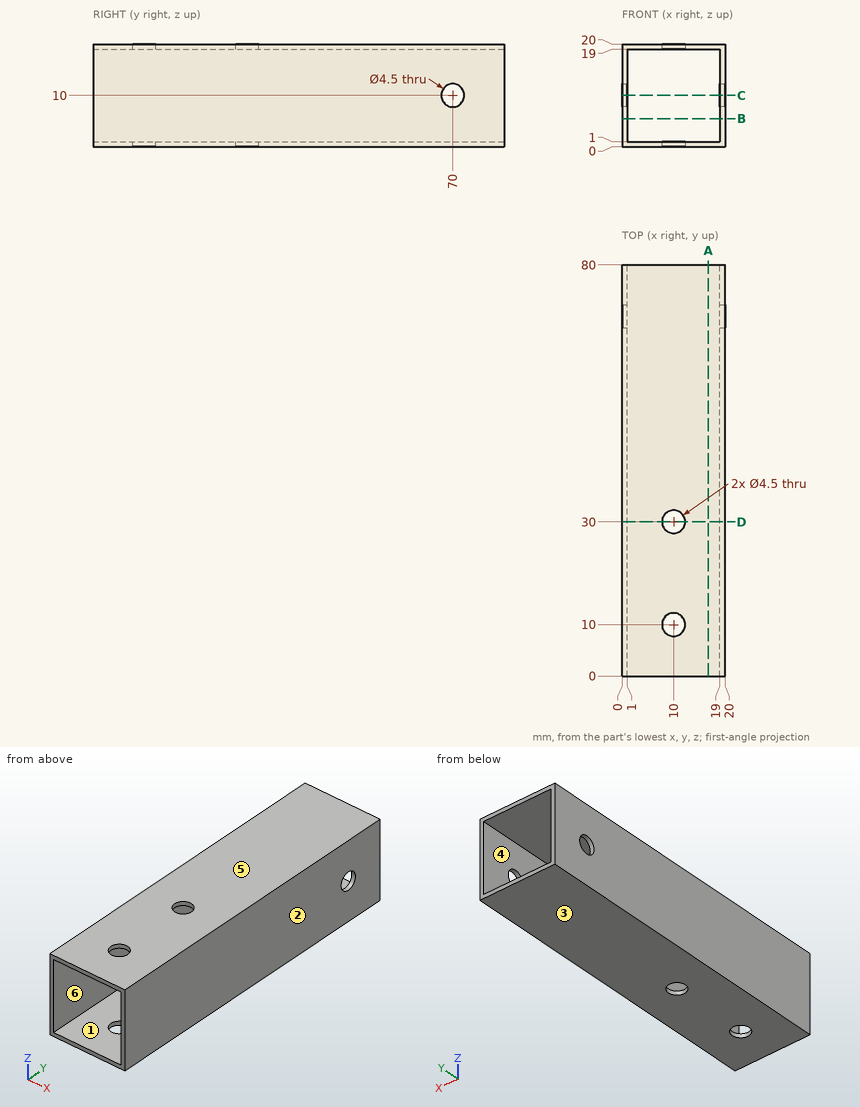
Check sheet for the drawn part. Datum: minimum x, y, z corner. Units: mm. A direction names the side the tool comes from. Round coordinates to 2 decimals unless told otherwise and drop trailing zeros. Order: outer loops, then holes, each group sorted by start corner. A loop starts at its lowest first (then second) coordinate and runs counter-clockwise, first axis right, second up.
1) Scan lines: line 1 (Y direction, x = 10, z = 0.5); line 2 (Z direction, x = 11.75, y = 66.5). Record each from-to range of solid material in increasing order.
2) Tool access check on the marked faces 1 and 2. Record the directions out of +Z, -Z, +X, -X, +Y, -Y that give a thin tool (end or side, any length) a straight path to the whole face; none if there is none.
3) Go/stop test with a flat-tipped pin: pin 1 Ø6 at (x, y) = (7.5, 41) entering from -Z. Record where the tip stops, or that it passes through.
4) Section check B-B (z = 5.5). Record the boundary of the cut face in (x, y).
5) Section check D-D (y = 30). Record the boundary of the cut face in (x, z), and give its area (3 significant figures).
6) Section check C-C (z = 10). Record the boundary of the cut face in (x, y).
7) Section check A-A (x = 16.75). Record the boundary of the cut face in (y, z).
8) Mould release check, pull along Z, two halves, no side actions. Record for the marked faces 3, 4, 5 and 6: +Z half, -Z half, draft (parallel to the pull), parting line (faces both ways), or undercut.
Result:
1. line 1: y = 0 to 7.75, 12.25 to 27.75, 32.25 to 80
1. line 2: z = 0 to 1, 19 to 20
2. face 1: +Y, -Y
2. face 2: +Z, -Z, +X, +Y, -Y
3. pin 1: stops at z = 0
4. outline: (0, 0) - (1, 0) - (1, 80) - (0, 80) - close; (19, 0) - (20, 0) - (20, 80) - (19, 80) - close
5. outline: (0, 0) - (7.75, 0) - (7.75, 1) - (1, 1) - (1, 19) - (7.75, 19) - (7.75, 20) - (0, 20) - close; (12.25, 0) - (20, 0) - (20, 20) - (12.25, 20) - (12.25, 19) - (19, 19) - (19, 1) - (12.25, 1) - close
5. area: 67.0 mm2
6. outline: (0, 0) - (1, 0) - (1, 67.75) - (0, 67.75) - close; (0, 72.25) - (1, 72.25) - (1, 80) - (0, 80) - close; (19, 0) - (20, 0) - (20, 67.75) - (19, 67.75) - close; (19, 72.25) - (20, 72.25) - (20, 80) - (19, 80) - close
7. outline: (0, 0) - (80, 0) - (80, 1) - (0, 1) - close; (0, 19) - (80, 19) - (80, 20) - (0, 20) - close
8. face 3: -Z half
8. face 4: undercut
8. face 5: +Z half
8. face 6: undercut
